Read the model definition and answer for the solid it produces. Units are mm, in the model's axes. A direction names the side the tool comes from. Round coordinates to 2 decimals unless told otherwise and drop trailing zeros. Write each loop counter-clockwise with the first axis right and the second up, starting at its lowest first coordinate (ties: lowest second). Pieces come first, ordered by that corner, then holes. Notation, with made-up numbers: (41.25, 61.5) - (89.25, 61.5) arc R23 cw to (89.25, 85.5) - close; hole circle Ø6 at (-39, 52). An arc over 180 degrees is marked (long way). One line per item, written item: value. Start each with the question number.
(1) Flat-ended cylindrical pins translate along their axes: pin 1 Ø5 at (x, y) = (16.5, 41.5) entering from -Z; pin 2 Ø1.5 at (x, z) = (-21.5, 1.5) entering from -Y; pin 3 Ø1.5 at (y, z) = (-5, 1) entering from +X. Find the tip coordinate at first contact, or state that the pin passes through.
(2) Find the intervals of material crossed by L1, parallel to Y at x = 0, z = 1.3; L2, parallel to Y at x = 15, z = 1.75; L3, parallel to X at y = -9, z = 0.65, in increasing order.
(3) A cutting plane is placed at D-D, the plane y = 41. Determine the outline of the cut face in (x, z).
(4) For faces 1 (the face through (-21, 26, 2)), 2 (the face through (12.5, -3, 2)), 3 (the face through (-0.208, -19.914, 2.465)), determine the directions among +Z, -Z, +X, -X, +Y, -Y from which every point of the face is accessible in a straight line to the end or side of a thin tool.
(5) A cutting plane is placed at B-B, the plane y = 3.5. Determine the outline of the cut face in (x, z).
(6) A cutting plane is placed at C-C, the plane z = 0.75. Determine the outline of the cut face in (x, y).
(7) A cutting plane is placed at A-A, the plane x = 0. Determine the outline of the cut face in (y, z).
(8) The mould has two halves that part along X. Classify faces 4 (the face through (-25, 51, 2)), 5 (the face through (-16.27, 40.03, 2.46)), 6 (the face through (1.526, 3.981, 2.465)), 7 (the face through (23, 78, 2)): +X half, -X half, draft (parallel to the pull), parting line (faces both ways), or undercut.
from build123d import *

# Parameters (mm, degrees)
SKETCH1_R           = 1.6
BOSS_EXTRUDE1_DEPTH = 5
FILLET1_R           = 5


with BuildPart() as part:
    # Sketch1 → Boss-Extrude1 (new body)
    with BuildSketch(Plane.XY):
        Polygon((-12.5, 26), (-12.5, -26), (12.5, -26), (12.5, 26), (25, 26), (25, 76), (20, 81), (-20, 81), (-25, 76), (-25, 26), align=None)
        with Locations((0, -21.5)):
            Circle(SKETCH1_R, mode=Mode.SUBTRACT)
        with Locations((0, 3.5)):
            Circle(SKETCH1_R, mode=Mode.SUBTRACT)
        with Locations((-15, 71)):
            Circle(SKETCH1_R, mode=Mode.SUBTRACT)
        with Locations((15, 71)):
            Circle(SKETCH1_R, mode=Mode.SUBTRACT)
        with Locations((-15, 41)):
            Circle(SKETCH1_R, mode=Mode.SUBTRACT)
        with Locations((15, 41)):
            Circle(SKETCH1_R, mode=Mode.SUBTRACT)
    extrude(amount=BOSS_EXTRUDE1_DEPTH)

    # Fillet1
    fillet1_edges = [part.edges().sort_by_distance(p)[0] for p in [
        (-12.5, 26, 2.5),
        (12.5, 26, 2.5),
    ]]
    fillet(fillet1_edges, radius=FILLET1_R)


solid = part.part
Here are the results:
1. pin 1: z = 0
1. pin 2: y = 26
1. pin 3: x = 12.5
2. L1: -26 to -23.1, -19.9 to 1.9, 5.1 to 81
2. L2: 25.33 to 39.4, 42.6 to 69.4, 72.6 to 81
2. L3: -12.5 to 12.5
3. outline: (-25, 0) - (-16.6, 0) - (-16.6, 5) - (-25, 5) - close; (-13.4, 0) - (13.4, 0) - (13.4, 5) - (-13.4, 5) - close; (16.6, 0) - (25, 0) - (25, 5) - (16.6, 5) - close
4. face 1: +Z, -Z, -X, -Y
4. face 2: +Z, -Z, +X, -Y
4. face 3: +Z, -Z
5. outline: (-12.5, 0) - (-1.6, 0) - (-1.6, 5) - (-12.5, 5) - close; (1.6, 0) - (12.5, 0) - (12.5, 5) - (1.6, 5) - close
6. outline: (-25, 26) - (-17.5, 26) arc R5 cw to (-12.5, 21) - (-12.5, -26) - (12.5, -26) - (12.5, 21) arc R5 cw to (17.5, 26) - (25, 26) - (25, 76) - (20, 81) - (-20, 81) - (-25, 76) - close; hole circle Ø3.2 at (-15, 41); hole circle Ø3.2 at (-15, 71); hole circle Ø3.2 at (0, -21.5); hole circle Ø3.2 at (0, 3.5); hole circle Ø3.2 at (15, 41); hole circle Ø3.2 at (15, 71)
7. outline: (-26, 0) - (-23.1, 0) - (-23.1, 5) - (-26, 5) - close; (-19.9, 0) - (1.9, 0) - (1.9, 5) - (-19.9, 5) - close; (5.1, 0) - (81, 0) - (81, 5) - (5.1, 5) - close
8. face 4: -X half
8. face 5: undercut
8. face 6: undercut
8. face 7: +X half
